```python
from build123d import *

# Parameters (mm, degrees)
PAD_DEPTH          = 15
SKETCH001_R        = 3.25
POCKET_DEPTH       = 40
SKETCH002_R        = 2.75
POCKET001_DEPTH    = 20
POCKET001_FACE10_W = 53
POCKET001_FACE10_H = 15
PAD001_DEPTH       = 10
SKETCH003_W        = 10
SKETCH003_H        = 60
POCKET002_DEPTH    = 20
POCKET002_FACE11_W = 45.5
POCKET002_FACE11_H = 15
POCKET003_DEPTH    = 10
SKETCH004_R        = 2.25
POCKET004_DEPTH    = 100
SKETCH005_R        = 2.75
POCKET005_DEPTH    = 15
SKETCH006_W        = 27.5
SKETCH006_H        = 15
POCKET006_DEPTH    = 10
SKETCH007_R        = 2.75
POCKET007_DEPTH    = 15
SKETCH009_R        = 5
POCKET008_DEPTH    = 6


with BuildPart() as part:
    # Sketch → Pad (new body)
    with BuildSketch(Plane.XY):
        Polygon((-16.5, 56.5), (-16.5, 9), (-26.5, 9), (-26.5, -26.5), (26.5, -26.5), (26.5, 9), (16.5, 9), (16.5, 56.5), align=None)
    extrude(amount=PAD_DEPTH)

    # Sketch001 (on Face7 of Pad) → Pocket (cut)
    with BuildSketch(Plane.YZ.offset(16.5)):
        with Locations((46.5, 7.5)):
            Circle(SKETCH001_R)
    extrude(amount=-POCKET_DEPTH, mode=Mode.SUBTRACT)

    # Sketch002 (on Face4 of Pocket) → Pocket001 (cut)
    with BuildSketch(Plane.XY.offset(15)):
        with Locations((-16.5, 0)):
            Circle(SKETCH002_R)
    extrude(amount=-POCKET001_DEPTH, mode=Mode.SUBTRACT)

    # Pocket001 Face10 → Pad001 (add)
    with BuildSketch(Plane(origin=(0, -26.5, 7.5), x_dir=(-1, 0, 0), z_dir=(0, -1, 0))):
        Rectangle(POCKET001_FACE10_W, POCKET001_FACE10_H)
    extrude(amount=PAD001_DEPTH)

    # Sketch003 (on Face10 of Pad001) → Pocket002 (cut)
    with BuildSketch(Plane.XY.offset(15)):
        Rectangle(SKETCH003_W, SKETCH003_H)
    extrude(amount=-POCKET002_DEPTH, mode=Mode.SUBTRACT)

    # Pocket002 Face11 → Pocket003 (cut)
    with BuildSketch(Plane(origin=(26.5, -13.75, 7.5), x_dir=(0, -1, 0), z_dir=(1, 0, 0))):
        Rectangle(POCKET002_FACE11_W, POCKET002_FACE11_H)
    extrude(amount=-POCKET003_DEPTH, mode=Mode.SUBTRACT)

    # Sketch004 (on Face14 of Pocket003) → Pocket004 (cut)
    with BuildSketch(Plane.YZ.offset(16.5)):
        with Locations((-14.5, 7.5)):
            Circle(SKETCH004_R)
        with Locations((14.5, 7.5)):
            Circle(SKETCH004_R)
    extrude(amount=-POCKET004_DEPTH, mode=Mode.SUBTRACT)

    # Sketch005 (on Face1 of Pocket004) → Pocket005 (cut)
    with BuildSketch(Plane(origin=(-16.5, 0, 0), x_dir=(0, -1, 0), z_dir=(-1, 0, 0))):
        with Locations((-14.5, 7.5)):
            Circle(SKETCH005_R)
    extrude(amount=-POCKET005_DEPTH, mode=Mode.SUBTRACT)

    # Sketch006 (on Face9 of Pocket005) → Pocket006 (cut)
    with BuildSketch(Plane(origin=(-26.5, 0, 0), x_dir=(0, -1, 0), z_dir=(-1, 0, 0))):
        with Locations((22.75, 7.5)):
            Rectangle(SKETCH006_W, SKETCH006_H)
    extrude(amount=-POCKET006_DEPTH, mode=Mode.SUBTRACT)

    # Sketch007 (on Face11 of Pocket006) → Pocket007 (cut)
    with BuildSketch(Plane(origin=(-16.5, 0, 0), x_dir=(0, -1, 0), z_dir=(-1, 0, 0))):
        with Locations((14.5, 7.5)):
            Circle(SKETCH007_R)
    extrude(amount=-POCKET007_DEPTH, mode=Mode.SUBTRACT)

    # Sketch009 (on Face8 of Pocket007) → Pocket008 (cut)
    with BuildSketch(Plane.YZ.offset(16.5)):
        with Locations((-14.5, 7.5)):
            Circle(SKETCH009_R)
        with Locations((14.5, 7.5)):
            Circle(SKETCH009_R)
    extrude(amount=-POCKET008_DEPTH, mode=Mode.SUBTRACT)


solid = part.part
```
Check sheet for the modelled part. Datum: model origin and axes. Units: mm. A direction names the side the tool comes from. Round coordinates to 2 decimals unless told otherwise and drop trailing zeros. Loops run counter-clockwise (first coordinate to the right, second up) from the corner with the lowest first, then second, coordinate; pieces in that order, holes last. Notation, with made-up numbers: (80, -8) - (115, -8) arc R26 ccw to (115, 15) - close; hole circle Ø2 at (15, 18.25). An arc over 180 degrees is marked (long way). Answer as a JSON object with one key per item and string values. Group by question number.
Q1. Sectioned sample at C-C, the plane y = 14.5. Enter the section's corners in (x, z).
Q2. Mould release check, pull along X, two halves, no side actions. Record for faces 4 (the face through (-16.5, 33, 7)), 5 (the face through (0, -30, 8)), 6 (the face through (7.788, 16.646, 8.176)): released by +X, released by -X, zero draft, split by the parting line, or undercut.
Q3. Set-up check for faces 1 (the face through (-10.83, 16.682, 5.827)), 2 (the face through (-21, 9, 7)), 3 (the face through (-22, -9, 7)): record each of +Z, -Z, +X, -X, +Y, -Y from which the full face is reachable in a straight line by a thin tool's end or side.
Q4. Sectioned sample at A-A, the plane y = 0. Enter the section's corners in (x, z), plus the area to 4 significant figures.
Q5. Sectioned sample at B-B, the plane z = 13.5. Enter the section's corners in (x, y), plus the area to 3 significant figures.
Q6. Scan lines: line 1 along X through (y, z) = (-25, 1.5); line 2 along Z through (x, y) = (13.3, 14.5); line 3 along X through (y, z) = (6.5, 4). Record each from-to range of solid material in increasing order. Write a range as [from, to].
Q7. Gauge pin test, flat ends, axial feed: P1, Ø6, axis at y = 14.5, z = 7.5, coming from the +X side; P2, Ø3, axis at x = -19, z = 13, coming from the -Y side; P3, Ø1, axis at y = -23.5, z = 8, coming from the -X side. Record the tip position at first contact, or that the pin passes through.
Q8. Sectioned sample at D-D, the plane x = -12.5. Enter the section's corners in (y, z), plus the area to 3 significant figures.
Solution:
{
 "1": {"outline": "(-16.5, 0) - (-5, 0) - (-5, 4.75) - (-16.5, 4.75) - close; (-16.5, 10.25) - (-5, 10.25) - (-5, 15) - (-16.5, 15) - close; (5, 0) - (16.5, 0) - (16.5, 2.5) - (10.5, 2.5) - (10.5, 5.25) - (5, 5.25) - close; (5, 9.75) - (10.5, 9.75) - (10.5, 12.5) - (16.5, 12.5) - (16.5, 15) - (5, 15) - close"},
 "2": {"face 4": "released by -X", "face 5": "undercut", "face 6": "zero draft"},
 "3": {"face 1": "-X", "face 2": "+Z, -Z, -X, +Y", "face 3": "+Z, -Z, -X, -Y"},
 "4": {"outline": "(-26.5, 0) - (-19.25, 0) - (-19.25, 15) - (-26.5, 15) - close; (-13.75, 0) - (-5, 0) - (-5, 15) - (-13.75, 15) - close; (5, 0) - (16.5, 0) - (16.5, 15) - (5, 15) - close", "area": "412.5 mm²"},
 "5": {"outline": "(-26.5, -9) - (-16.5, -9) - (-16.5, -36.5) - (16.5, -36.5) - (16.5, 56.5) - (-16.5, 56.5) - (-16.5, 9) - (-26.5, 9) - close; hole circle Ø5.5 at (-16.5, 0); hole (-5, -30) - (5, -30) - (5, 30) - (-5, 30) - close", "area": "2,630 mm²"},
 "6": {"line 1": "x = [-16.5, -5], [5, 16.5]", "line 2": "z = [0, 2.5], [12.5, 15]", "line 3": "x = [-26.5, -5], [5, 16.5]"},
 "7": {"P1": "stops at x = 10.5", "P2": "stops at y = -9", "P3": "stops at x = -16.5"},
 "8": {"outline": "(-36.5, 0) - (56.5, 0) - (56.5, 15) - (-36.5, 15) - close; hole circle Ø5.5 at (-14.5, 7.5); hole circle Ø5.5 at (14.5, 7.5); hole circle Ø6.5 at (46.5, 7.5)", "area": "1,310 mm²"}
}
